```python
from build123d import *

# Parameters (mm, degrees)
SKETCH1_R           = 2.54
SKETCH1_R_2         = 2.25
SKETCH1_R_3         = 1.75
SKETCH1_R_4         = 2.5
SKETCH1_R_5         = 11.5
BOSS_EXTRUDE1_DEPTH = 3
FILLET2_R           = 2.54


with BuildPart() as part:
    # Sketch1 → Boss-Extrude1 (new body)
    with BuildSketch(Plane.XY):
        with BuildLine():
            Line((0, 0), (0, -29.5))
            Line((0, -29.5), (-37, -29.5))
            ThreePointArc((-37, -29.5), (-38.114378278, -31.538839171), (-38.5, -33.830127019))
            Line((-38.5, -33.830127019), (-38.5, -44.16209895))
            ThreePointArc((-38.5, -44.16209895), (-42.014718626, -52.647380324), (-50.5, -56.16209895))
            Line((-50.5, -56.16209895), (-84.414235636, -56.16209895))
            ThreePointArc((-84.414235636, -56.16209895), (-90.428351627, -55.236437965), (-95.885764364, -52.545139836))
            Line((-95.885764364, -52.545139836), (-121.385764364, -34.689847611))
            ThreePointArc((-121.385764364, -34.689847611), (-124.520108332, -31.115813301), (-125.65, -26.498327168))
            Line((-125.65, -26.498327168), (-125.65, 7.501672832))
            ThreePointArc((-125.65, 7.501672832), (-124.809828805, 11.670050653), (-122.420515459, 15.187499024))
            Line((-122.420515459, 15.187499024), (-97.551844693, 35.325751537))
            ThreePointArc((-97.551844693, 35.325751537), (-84.833866838, 36.831023412), (-78, 26))
            Line((-78, 26), (-78, 13))
            ThreePointArc((-78, 13), (-74.192388155, 3.807611845), (-65, 0))
            Line((-65, 0), (0, 0))
        make_face()
        with Locations((-18.237, -9.806)):
            Circle(SKETCH1_R, mode=Mode.SUBTRACT)
        with Locations((-48.5, -9.75)):
            Circle(SKETCH1_R_2, mode=Mode.SUBTRACT)
        with Locations((-74.5, -9.75)):
            Circle(SKETCH1_R_2, mode=Mode.SUBTRACT)
        with Locations((-89, 5.6)):
            Circle(SKETCH1_R_3, mode=Mode.SUBTRACT)
        with Locations((-89, 25.5)):
            Circle(SKETCH1_R_4, mode=Mode.SUBTRACT)
        with Locations((-89, -25.1)):
            Circle(SKETCH1_R_3, mode=Mode.SUBTRACT)
        with Locations((-89, -45.112)):
            Circle(SKETCH1_R_4, mode=Mode.SUBTRACT)
        with Locations((-104.35, -9.75)):
            Circle(SKETCH1_R_5, mode=Mode.SUBTRACT)
        with Locations((-119.7, 5.6)):
            Circle(SKETCH1_R_3, mode=Mode.SUBTRACT)
        with Locations((-119.7, -25.1)):
            Circle(SKETCH1_R_3, mode=Mode.SUBTRACT)
    extrude(amount=BOSS_EXTRUDE1_DEPTH)

    # Fillet2
    fillet2_edges = [part.edges().sort_by_distance(p)[0] for p in [
        (0, 0, 1.5),
        (0, -29.5, 1.5),
    ]]
    fillet(fillet2_edges, radius=FILLET2_R)


solid = part.part
```
Geometry check sheet. Reference: the model listing, model coordinates, mm. A direction names the side the tool comes from. Give positions to 0.01 mm unless a question says otherwise; leave off trailing zeros. Write each loop counter-clockwise with the first axis right and the second up, starting at its lowest first coordinate (ties: lowest second). Pieces come first, ordered by that corner, then holes.
1) Gauge pin test, flat ends, axial feed: pin 1 (1.5 mm diameter, centred on x = -24.5, z = 1, fed in from +Y); pin 2 (1.5 mm diameter, centred on y = 16.5, z = 1, fed in from +X); pin 3 (1.5 mm diameter, centred on x = -18, z = 1.5, fed in from -Y). Record the tip position at first contact, or that the pin passes through.
2) Access from +Z, -Z, +X, -X, +Y, -Y to the whole of each face (thin tool, end or side, straight path). Record for faces 5 (the flat face through (-34, 0, 1)), 6 (the flat face through (-38.5, -39, 1)), 7 (the flat face through (-67, -56.162, 1)).
3) Section check B-B, the plane y = -25.1. Record the boundary of the cut face in (x, z), and give its area (3 significant figures).
4) Section check A-A, the plane x = -89. Record the boundary of the cut face in (y, z), and give its area (3 significant figures).
5) Material ranges on L1, parallel to X at y = -9, z = 0.35; L2, parallel to Y at x = -89, z = 1.5; L3, parallel to X at y = 6, z = 1.1, recorded low to high.
6) Release check for a two-part mould opening along X. For faces 1 (the cylindrical face through (-91, 27, 1)), 2 (the flat face through (-110.16, 25.116, 1.479)), 3 (the cylindrical face through (-74.293, 3.909, 1.479)), 4 (the cylindrical face through (-72.354, -9.074, 1.479)) record: pulls with the +X half, pulls with the -X half, needs draft (parallel to the pull), parting line crosses it, or undercut.
7) Section check C-C, the plane x = -104.35. Record the boundary of the cut face in (y, z), and give its area (3 significant figures).
8) Section check D-D, the plane z = 2.2. State how many separate pieces and enclosed holes the cut face has, and give its area (3 significant figures).
Computed:
1. pin 1: stops at y = 0
1. pin 2: stops at x = -78
1. pin 3: stops at y = -29.5
2. face 5: +Z, -Z, +X, +Y
2. face 6: +Z, -Z, +X, -Y
2. face 7: +Z, -Z, +X, -X, -Y
3. outline: (-125.65, 0) - (-121.45, 0) - (-121.45, 3) - (-125.65, 3) - close; (-117.95, 0) - (-90.75, 0) - (-90.75, 3) - (-117.95, 3) - close; (-87.25, 0) - (0, 0) - (0, 3) - (-87.25, 3) - close
3. area: 356 mm2
4. outline: (-55.63, 0) - (-47.61, 0) - (-47.61, 3) - (-55.63, 3) - close; (-42.61, 0) - (-26.85, 0) - (-26.85, 3) - (-42.61, 3) - close; (-23.35, 0) - (3.85, 0) - (3.85, 3) - (-23.35, 3) - close; (7.35, 0) - (23, 0) - (23, 3) - (7.35, 3) - close; (28, 0) - (37.96, 0) - (37.96, 3) - (28, 3) - close
4. area: 230 mm2
5. L1: x = -125.65 to -115.83, -92.87 to -76.62, -72.38 to -50.62, -46.38 to -20.65, -15.83 to 0
5. L2: y = -55.63 to -47.61, -42.61 to -26.85, -23.35 to 3.85, 7.35 to 23, 28 to 37.96
5. L3: x = -125.65 to -121.4, -118 to -90.7, -87.3 to -75.95
6. face 1: undercut
6. face 2: pulls with the -X half
6. face 3: pulls with the +X half
6. face 4: undercut
7. outline: (-46.62, 0) - (-21.25, 0) - (-21.25, 3) - (-46.62, 3) - close; (1.75, 0) - (29.82, 0) - (29.82, 3) - (1.75, 3) - close
7. area: 160 mm2
8. separate pieces: 1
8. enclosed holes: 10
8. area: 6,430 mm2
